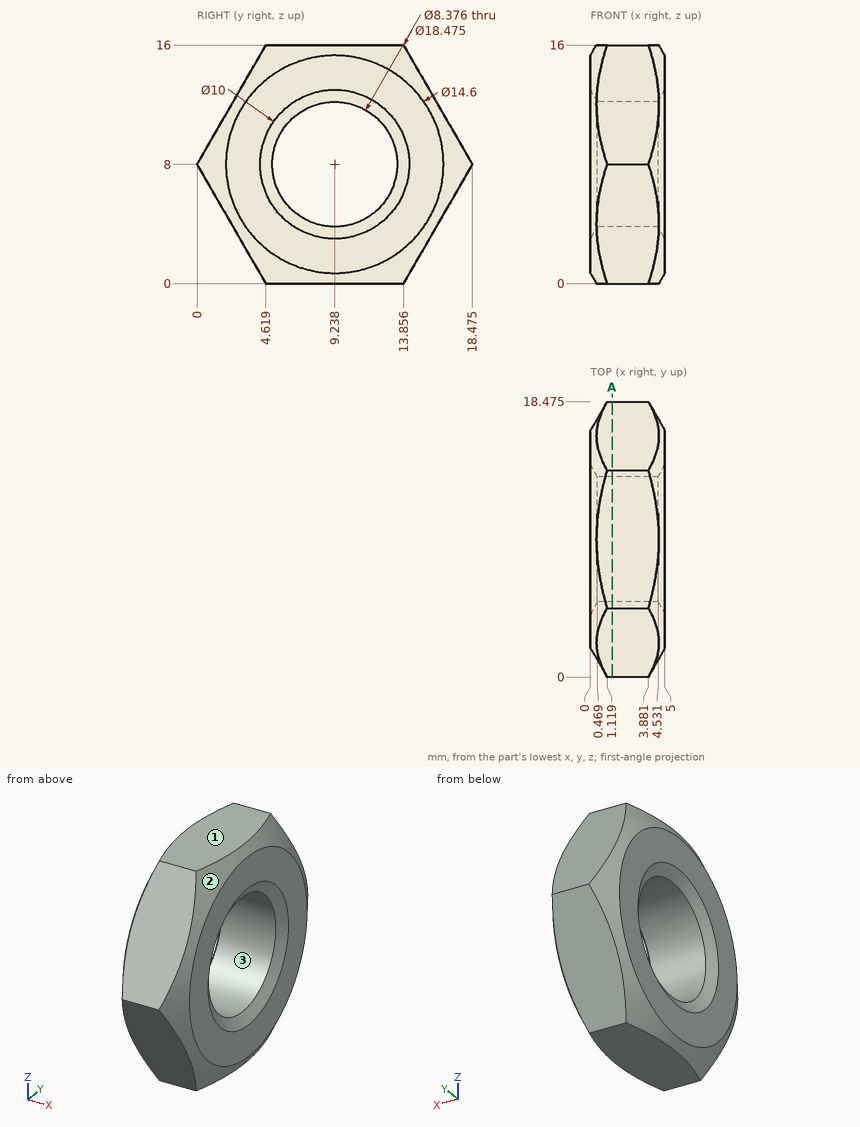
Geometry check sheet. Reference: drawing and pictorial views, mm from the part's lowest x, y, z. Give positions to 0.01 mm unless a question says otherwise; leave off trailing zeros. Write each loop counter-clockwise with the first axis right and the second up, starting at its lowest first coordinate (ties: lowest second). Pieces come first, ordered by that corner, then holes. Notation, with made-up numbers: (50, 58) - (101, 58) arc R23 ccw to (101, 84) - close; hole circle Ø10 at (57, 37). An arc over 180 degrees is marked (long way). Put each result on its own line as item: value.
Q1. Mould release check, pull along Y, two halves, no side actions. Record for the marked faces 1, 2 and 3: released by +Y, released by -Y, zero draft, split by the parting line, or undercut.
Result:
face 1: zero draft
face 2: split by the parting line
face 3: undercut
Q2. Scan lines: probe 1 along Y at (x, z) = (2.55, 10.75) (1 decimal); probe 2 along Y at (x, z) = (2.25, 7.5) (1 decimal); probe 3 along Z at (x, y) = (4.65, 11.5) (1 decimal). Record each from-to range of solid material in increasing order. Write a range as from..to.
Result:
probe 1: 1.6..6.1, 12.4..16.9
probe 2: 0.3..5.1, 13.4..18.2
probe 3: 0.4..4.2, 11.8..15.6
Q3. Depth check by flat-ended pin: P1, Ø1, axis at y = 3.5, z = 3, coming from the +X side. Enter the tip coordinate at first touch or a pass-through.
Result:
P1: x = 5
Q4. Section check A-A on x = 1.45. Record the cut outline in (y, z) (1 decimal).
Result:
outline: (0, 8) - (4.6, 0) - (13.9, 0) - (18.5, 8) - (13.9, 16) - (4.6, 16) - close; hole circle Ø8.4 at (9.2, 8)
